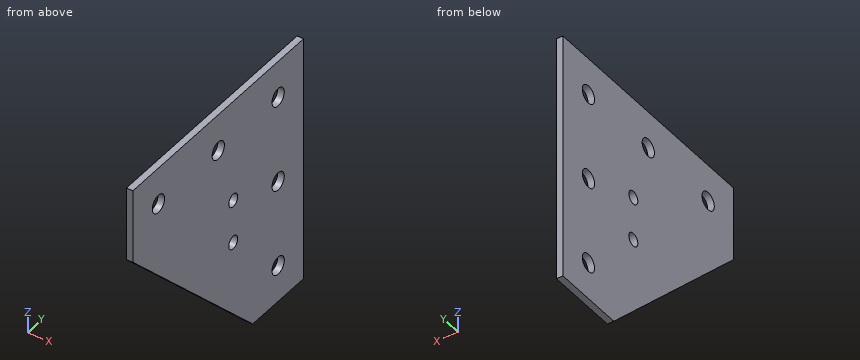
from build123d import *

# Parameters (mm, degrees)
SKETCH_1_W          = 114
SKETCH_1_H          = 114
EXTRUDE_266_DEPTH   = 3
SKETCH_2_R          = 4.1
CUT_EXTRUDE_1_DEPTH = 81.665977958
CUT_EXTRUDE_2_DEPTH = 81.665977958
SKETCH_4_R          = 3
CUT_EXTRUDE_3_DEPTH = 81.665977958


with BuildPart() as part:
    # Эскиз1 → Extrude 266 (new body)
    with BuildSketch(Plane(origin=(0, 0, 0), x_dir=(0, 0, -1), z_dir=(1, 0, 0))):
        Rectangle(SKETCH_1_W, SKETCH_1_H)
    extrude(amount=EXTRUDE_266_DEPTH)

    # Эскиз2 → Вырез-Вытянуть1 (cut, through all)
    with BuildSketch(Plane(origin=(3, 0, 0), x_dir=(0, 0, -1), z_dir=(1, 0, 0))):
        with Locations((0, 40)):
            Circle(SKETCH_2_R)
        with Locations((40, 40)):
            Circle(SKETCH_2_R)
        with Locations((-40, 0)):
            Circle(SKETCH_2_R)
        with Locations((-40, -40)):
            Circle(SKETCH_2_R)
        with Locations((-40, 40)):
            Circle(SKETCH_2_R)
    extrude(amount=-CUT_EXTRUDE_1_DEPTH, mode=Mode.SUBTRACT)

    # Эскиз3 → Вырез-Вытянуть2 (cut, through all)
    with BuildSketch(Plane(origin=(3, 0, 0), x_dir=(0, 0, -1), z_dir=(1, 0, 0))):
        Polygon((57, 23), (57, -57), (-23, -57), align=None)
    extrude(amount=-CUT_EXTRUDE_2_DEPTH, mode=Mode.SUBTRACT)

    # Эскиз4 → Вырез-Вытянуть3 (cut, through all)
    with BuildSketch(Plane(origin=(3, 0, 0), x_dir=(0, 0, -1), z_dir=(1, 0, 0))):
        with Locations((-10, 10)):
            Circle(SKETCH_4_R)
        with Locations((10, 10)):
            Circle(SKETCH_4_R)
    extrude(amount=-CUT_EXTRUDE_3_DEPTH, mode=Mode.SUBTRACT)


solid = part.part
Read the model definition and answer for the solid it produces. Units are mm, in the model's axes. Give positions to 0.01 mm unless a question says otherwise; leave off trailing zeros. Write each loop counter-clockwise with the first axis right and the second up, starting at its lowest first coordinate (ties: lowest second). Pieces come first, ordered by that corner, then holes. Notation, with made-up numbers: (-12.75, -19) - (-0.75, -19) arc R15 cw to (-0.75, 8) - close; hole circle Ø6 at (85.25, 33). An arc over 180 degrees is marked (long way). Use CSV: the item, a comma, the result in double quotes. Start each with the question number.
(1) Find section D-D (y = 19). Give the vertices of the cut face in (x, z).
(2) Find section B-B (z = 10). Give the vertices of the cut face in (x, y), plus the area to 3 significant figures.
(3) Find section A-A (y = -40). Give the vertices of the cut face in (x, z), plus the area to 3 significant figures.
(4) Find section C-C (x = 2.2). Give the vertices of the cut face in (y, z).
(5) Given P1, Ø9.5, axis at y = 10, z = 10, coming from the +X side, flat-ended and moving along its own axis, determine where the tip first touches the part or whether it passes through.
(6) Consider line 1 along Y through (x, z) = (2, 40); line 2 along Y through (x, z) = (1.1, 42.5); line 3 along Y through (x, z) = (0.65, -40). Determine where each line is inside the solid, lowest interval first.
Findings below:
1,outline,"(0, -53) - (3, -53) - (3, 57) - (0, 57) - close"
2,outline,"(0, -44) - (3, -44) - (3, 7) - (0, 7) - close; (0, 13) - (3, 13) - (3, 57) - (0, 57) - close"
2,area,"285 mm2"
3,outline,"(0, 6) - (3, 6) - (3, 35.9) - (0, 35.9) - close; (0, 44.1) - (3, 44.1) - (3, 57) - (0, 57) - close"
3,area,"128 mm2"
4,outline,"(-57, 23) - (23, -57) - (57, -57) - (57, 57) - (-57, 57) - close; hole circle Ø8.2 at (-40, 40); hole circle Ø8.2 at (0, 40); hole circle Ø6 at (10, -10); hole circle Ø6 at (10, 10); hole circle Ø8.2 at (40, -40); hole circle Ø8.2 at (40, 0); hole circle Ø8.2 at (40, 40)"
5,P1,"x = 3"
6,line 1,"-57 to -44.1, -35.9 to -4.1, 4.1 to 35.9, 44.1 to 57"
6,line 2,"-57 to -43.25, -36.75 to -3.25, 3.25 to 36.75, 43.25 to 57"
6,line 3,"6 to 35.9, 44.1 to 57"
